Autodesk Inventor part; units mm, degrees
ref_plane "YZ Plane" through (0, 0, 0) normal (1, 0, 0) x (0, 1, 0)
ref_plane "XZ Plane" through (0, 0, 0) normal (0, 1, 0) x (-1, 0, 0)
ref_plane "XY Plane" through (0, 0, 0) normal (0, 0, 1) x (1, 0, 0)
sketch "Sketch1" plane through (0, 0, 0) normal (0, 0, 1) x (1, 0, 0)
  line L0 (-69.9828, 73.1946) -> (155.0172, 73.1946)
  line L1 (155.0172, 73.1946) -> (155.0172, 43.1946)
  line L2 (155.0172, 43.1946) -> (-69.9828, 43.1946)
  line L3 (-69.9828, 43.1946) -> (-69.9828, 73.1946)
  line L4 (-69.9828, 73.1946) -> (-69.9828, 143.1946)
  line L5 (-69.9828, 143.1946) -> (155.0172, 73.1946)
  line L6 (-74.9828, 93.1946) -> (-74.9828, 38.1946)
  line L7 (-74.9828, 38.1946) -> (160.0172, 38.1946)
  line L8 (160.0172, 38.1946) -> (160.0172, 76.8754)
  line L9 (-74.9828, 73.1946) -> (-74.9828, 149.9865)
  line L10 (-74.9828, 149.9865) -> (160.0172, 76.8754)
  line L11 (-69.9828, 143.1946) -> (-74.9828, 143.1946)
  line L12 (155.0172, 73.1946) -> (160.0172, 73.1946)
  line L13 (-69.9828, 73.1946) -> (-74.9828, 73.1946)
  point P0 (0, 0)
  point P1 (-74.9828, 93.1946)
  dimension "d0" = 225
  dimension "d1" = 30
  dimension "d2" = 70
  dimension "d3" = 5
  dimension "d4" = 5
  dimension "d32" = 5
extrude "Extrusion1" add sketch "Sketch1" along normal blind 340 contours L13 L6 L9 L11 L4 | L3 L2 L1 L12 L8 L7 L6 L13 | L5 L11 L9 L10 L8 L12
extrude "Extrusion2" add sketch "Sketch1" along normal blind 340 contours L4 L5 L0 | L0 L1 L2 L3
extrude "Extrusion3" cut sketch "Sketch1" along normal blind 335 contours L4 L5 L0 | L0 L1 L2 L3
extrude "Extrusion4" add sketch "Sketch1" along normal blind 5 contours L4 L5 L0 | L0 L1 L2 L3
sketch "Sketch2" plane through (-74.9828, 149.9865, 340) normal (0.2971, 0.9549, 0) x (0.9549, -0.2971, 0)
  line L0 (36.4986, 335) -> (36.4986, 5)
  circle A0 centre (36.4986, 75.4833) radius 7.5
  circle A1 centre (53.1004, 265.9353) radius 10
  circle A2 centre (108.208, 107.2253) radius 10
  circle A3 centre (63.1004, 176.4405) radius 10
  circle A4 centre (158.9071, 36.2466) radius 7.5
  circle A5 centre (180.5093, 255.9353) radius 10
  circle A6 centre (144.7995, 198.4836) radius 10
  circle A7 centre (195.4985, 117.2253) radius 10
  point P0 (116.1538, 340)
  dimension "d13" = 15
  dimension "d14" = 20
  dimension "d15" = 20
  dimension "d16" = 20
  dimension "d17" = 15
  dimension "d18" = 20
  dimension "d19" = 20
  dimension "d20" = 20
extrude "Extrusion5" add sketch "Sketch2" along normal blind 5
sketch "Sketch3" plane through (0, 0, 340) normal (0, 0, 1) x (1, 0, 0)
  line L0 (-69.9828, 143.1946) -> (158.5319, 72.1011)
  line L1 (160.0172, 76.8754) -> (-74.9828, 149.9865)
  line L2 (-75.9241, 124.0974) -> (155.0172, 52.249)
  line L3 (-69.9828, 143.1946) -> (-69.9828, 122.249)
  line L4 (-69.9828, 43.1946) -> (-69.9828, 143.1946)
  line L5 (155.0172, 43.1946) -> (155.0172, 73.1946)
  line L6 (155.0172, 73.1946) -> (155.0172, 52.249)
  line L7 (-74.9828, 149.9865) -> (-74.9828, 174.9865)
  line L8 (-74.9828, 174.9865) -> (160.0172, 101.8754)
  line L9 (-69.9828, 143.1946) -> (155.0172, 73.1946)
  line L10 (160.0172, 76.8754) -> (160.0172, 101.8754)
  line L11 (-77.4095, 119.3231) -> (160.0172, 45.4571)
  line L12 (160.0172, 45.4571) -> (160.0172, 93.1946)
  line L13 (-69.9828, 122.249) -> (-69.9828, 117.0126)
  line L14 (155.0172, 52.249) -> (155.0172, 47.0126)
  point P0 (0, 0)
  dimension "d23" = 20
  dimension "d24" = 25
  dimension "d25" = 5
extrude "Extrusion6" add sketch "Sketch3" against normal blind 340 contours L2 L5 L11 L4
extrude "Extrusion7" add sketch "Sketch3" against normal blind 5 contours L1 L7 L8 L10
sketch "Sketch4" plane through (0, 0, 0) normal (0, 0, -1) x (-1, 0, 0)
  line L0 (74.9828, 174.9865) -> (74.9828, 38.1946)
  line L1 (74.9828, 169.9638) -> (74.9828, 174.9865)
  line L2 (-160.0172, 38.1946) -> (-160.0172, 101.8754)
  line L3 (74.9828, 174.9865) -> (-160.0172, 101.8754)
  line L4 (-160.0172, 101.8754) -> (-160.0172, 91.5878)
  line L5 (-160.0172, 76.8754) -> (74.9828, 149.9865)
  line L6 (74.9828, 149.9865) -> (-160.0172, 76.8754)
  point P0 (0, 0)
extrude "Extrusion8" add sketch "Sketch4" against normal blind 5
properties part number "newcollection"
The listing builds one solid part. Answer for the finished solid, in the listing's coordinates (mm). A direction names the side the tool comes from. Round coordinates to 2 decimals unless told otherwise and drop trailing zeros. Loops run counter-clockwise (first coordinate to the right, second up) from the corner with the lowest first, then second, coordinate; pieces in that order, holes last.
1) Given P1, Ø2, axis at x = -48.5, z = 77, coming from the +Y side; P2, Ø3, axis at x = 109, z = 45, coming from the +Y side, each flat-ended and moving along its own axis, determine where each tip first touches the part or whether it passes through.
Outcome:
P1: stops at y = 142.06
P2: stops at y = 93.21
2) For faces 4 (the face through (40.872, 138.943, 2.465)), 5 (the face through (44, 43.195, 168)), 6 (the face through (113.041, 96.723, 222.635)), determine the directions among +Z, -Z, +X, -X, +Y, -Y from which every point of the face is accessible in a straight line to the end or side of a thin tool.
Outcome:
face 4: +Z, -Z, +X, +Y
face 5: none
face 6: +X, +Y
3) Consider line 1 (Z direction, x = 48.5, y = 58); line 2 (Y direction, x = 126, z = 74); line 3 (Y direction, x = 22, z = 298). Determine where each line is inside the solid, lowest interval first.
Outcome:
line 1: z = 0 to 5, 335 to 340
line 2: y = 38.19 to 43.19, 56.04 to 61.28, 82.22 to 87.46
line 3: y = 38.19 to 43.19, 88.4 to 93.63, 114.58 to 119.81
4) For a pull along Z with two mould halves and no side action, classify faces 1 (the face through (15, 92, 340)), 2 (the face through (-16.1, 134.2, 153.8)), 3 (the face through (-74.983, 92, 168)) as released by +Z, released by -Z, zero draft, split by the parting line, or undercut.
Outcome:
face 1: released by +Z
face 2: undercut
face 3: zero draft
5) A cutting plane is placed at A-A on x = 129.5. Determine the outline of the cut face in (y, z).
Outcome:
outline: (38.19, 0) - (111.37, 0) - (111.37, 5) - (86.37, 5) - (86.37, 335) - (111.37, 335) - (111.37, 340) - (38.19, 340) - close; hole (43.19, 5) - (54.95, 5) - (54.95, 335) - (43.19, 335) - close; hole (60.19, 5) - (81.13, 5) - (81.13, 335) - (60.19, 335) - close
6) A cutting plane is placed at B-B on y = 154.5. Determine the outline of the cut face in (x, z), plus the area to 3 significant figures.
Outcome:
outline: (-74.98, 0) - (-9.13, 0) - (-9.13, 5) - (-74.98, 5) - close; (-74.98, 335) - (-9.13, 335) - (-9.13, 340) - (-74.98, 340) - close
area: 658 mm2
7) A cutting plane is placed at D-D on z = 283. Determine the outline of the cut face in (x, y), plus the area to 3 significant figures.
Outcome:
outline: (-74.98, 38.19) - (160.02, 38.19) - (160.02, 76.88) - (-74.98, 149.99) - close; hole (-69.98, 43.19) - (155.02, 43.19) - (155.02, 47.01) - (-69.98, 117.01) - close; hole (-69.98, 122.25) - (155.02, 52.25) - (155.02, 73.19) - (-69.98, 143.19) - close
area: 4,230 mm2
8) A cutting plane is placed at C-C on z = 217. Determine the outline of the cut face in (x, y).
Outcome:
outline: (-74.98, 38.19) - (160.02, 38.19) - (160.02, 76.88) - (119.49, 89.49) - (120.97, 94.26) - (105.38, 99.11) - (103.89, 94.34) - (-74.98, 149.99) - close; hole (-69.98, 43.19) - (155.02, 43.19) - (155.02, 47.01) - (-69.98, 117.01) - close; hole (-69.98, 122.25) - (155.02, 52.25) - (155.02, 73.19) - (-69.98, 143.19) - close
